Geometry check sheet. Reference: drawing and pictorial views, mm from the part's lowest x, y, z. A direction names the side the tool comes from. Coordinates: 2 decimals unless noted, no trailing zeros. Loops run counter-clockwise (first coordinate to the right, second up) from the corner with the lowest first, then second, coordinate; pieces in that order, holes last.
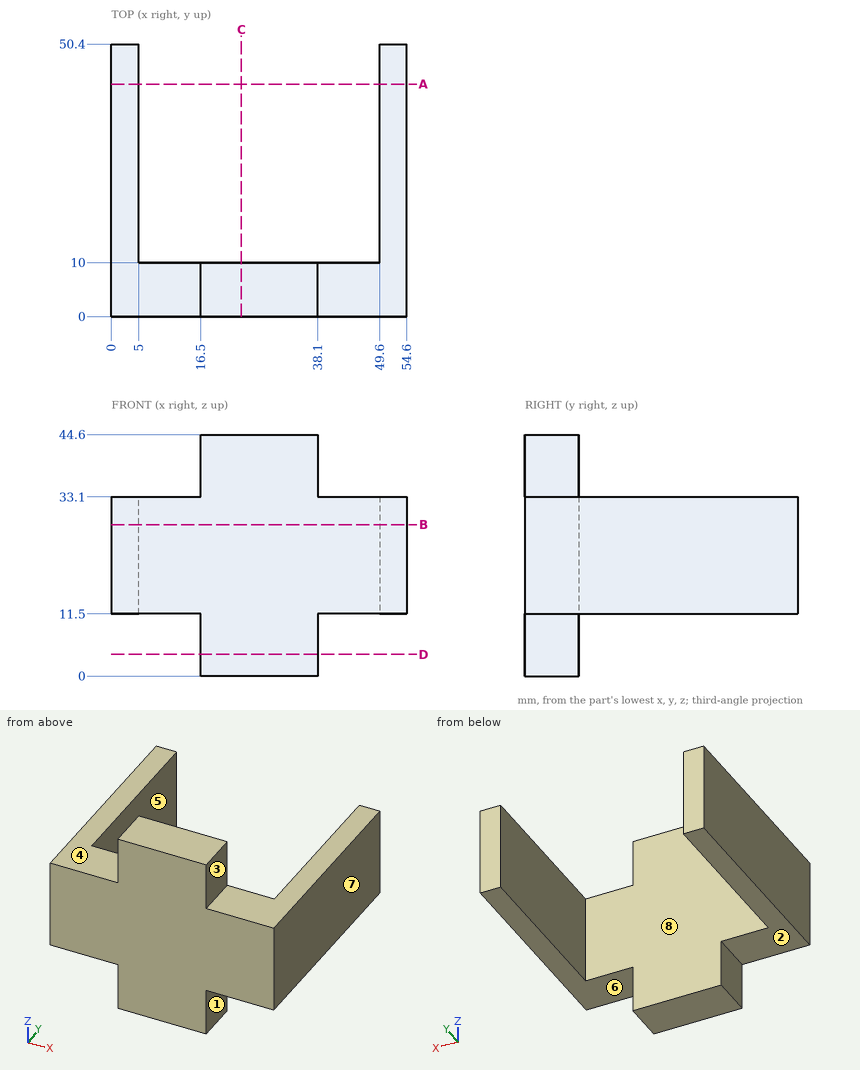
1) Depth check by flat-ended pin: pin 1 (5 mm diameter, centred on x = 12.5, z = 11, fed in from -Y); pin 2 (12 mm diameter, centred on x = 8, y = 11.5, fed in from +Z); pin 3 (3 mm diameter, centred on y = 6, z = 5, fed in from +X); pin 4 (3 mm diameter, centred on y = 3.5, z = 4, fed in from -X). Enter the tip coordinate at first touch or a pass-through.
Data:
pin 1: stops at y = 0
pin 2: stops at z = 33.1
pin 3: stops at x = 38.1
pin 4: stops at x = 16.5
2) Mould release check, pull along X, two halves, no side actions. Record for the marked faces 6, 7 and 8: +X half, -X half, draft (parallel to the pull), parting line (faces both ways), or undercut.
Data:
face 6: draft
face 7: +X half
face 8: undercut
3) Access from +Z, -Z, +X, -X, +Y, -Y to the whole of each face (thin tool, end or side, straight path). Record for the marked faces 1, 2, 3, 4 and 5.
Data:
face 1: -Z, +X, +Y, -Y
face 2: -Z, -X, +Y, -Y
face 3: +Z, +X, +Y, -Y
face 4: +Z, -X, +Y, -Y
face 5: +Z, -Z, +Y
4) Section check A-A on y = 43. Record the cut outline in (x, z).
Data:
outline: (0, 11.5) - (5, 11.5) - (5, 33.1) - (0, 33.1) - close; (49.6, 11.5) - (54.6, 11.5) - (54.6, 33.1) - (49.6, 33.1) - close
5) Section check B-B on z = 28. Record the cut outline in (x, y).
Data:
outline: (0, 0) - (54.6, 0) - (54.6, 50.4) - (49.6, 50.4) - (49.6, 10) - (5, 10) - (5, 50.4) - (0, 50.4) - close
6) Material ranges on probe 1 along X at (y, z) = (21, 33); probe 2 along Z at (x, y) = (2, 4); probe 3 along Y at (x, z) = (26, 39.5), recorded low to high.
Data:
probe 1: x = 0 to 5, 49.6 to 54.6
probe 2: z = 11.5 to 33.1
probe 3: y = 0 to 10
7) Section check D-D on z = 4. Record the cut outline in (x, y).
Data:
outline: (16.5, 0) - (38.1, 0) - (38.1, 10) - (16.5, 10) - close
8) Section check C-C on x = 24. Record the cut outline in (y, z).
Data:
outline: (0, 0) - (10, 0) - (10, 44.6) - (0, 44.6) - close
